Check sheet for the drawn part. Datum: minimum x, y, z corner. Units: mm. Give positions to 0.01 mm unless a question says otherwise; leave off trailing zeros. Loops run counter-clockwise (first coordinate to the right, second up) from the corner with the lowest first, then second, coordinate; pieces in that order, holes last. Notation, with made-up numbers: (-16, 63) - (36, 63) arc R17 ccw to (36, 78) - close; hole circle Ø1 at (66.5, 33.5). An arc over 180 degrees is marked (long way). One line per item, written item: value. Start each with the question number.
1. Gauge pin test, flat end, axial feed: pin 1 (0.8 mm diameter, centred on y = 1, z = 100, fed in from -X). Record the tip position at first contact, or that the pin passes through.
2. Scan lines: L1, parallel to Z at x = 14.5, y = 0.5; L2, parallel to X at y = 1.05, z = 121; L3, parallel to Z at x = 51.5, y = 1.4. Record each from-to range of solid material in increasing order. Write a range as [from, to].
3. Sectioned sample at D-D (z = 83). Record the cut outline in (x, y), plus the area to 3 significant figures.
4. Sectioned sample at B-B (y = 0.6). Record the cut outline in (x, z).
5. Sectioned sample at A-A (x = 50.5). Record the cut outline in (y, z).
6. Sectioned sample at C-C (z = 121). Record the cut outline in (x, y), plus the area to 3 significant figures.
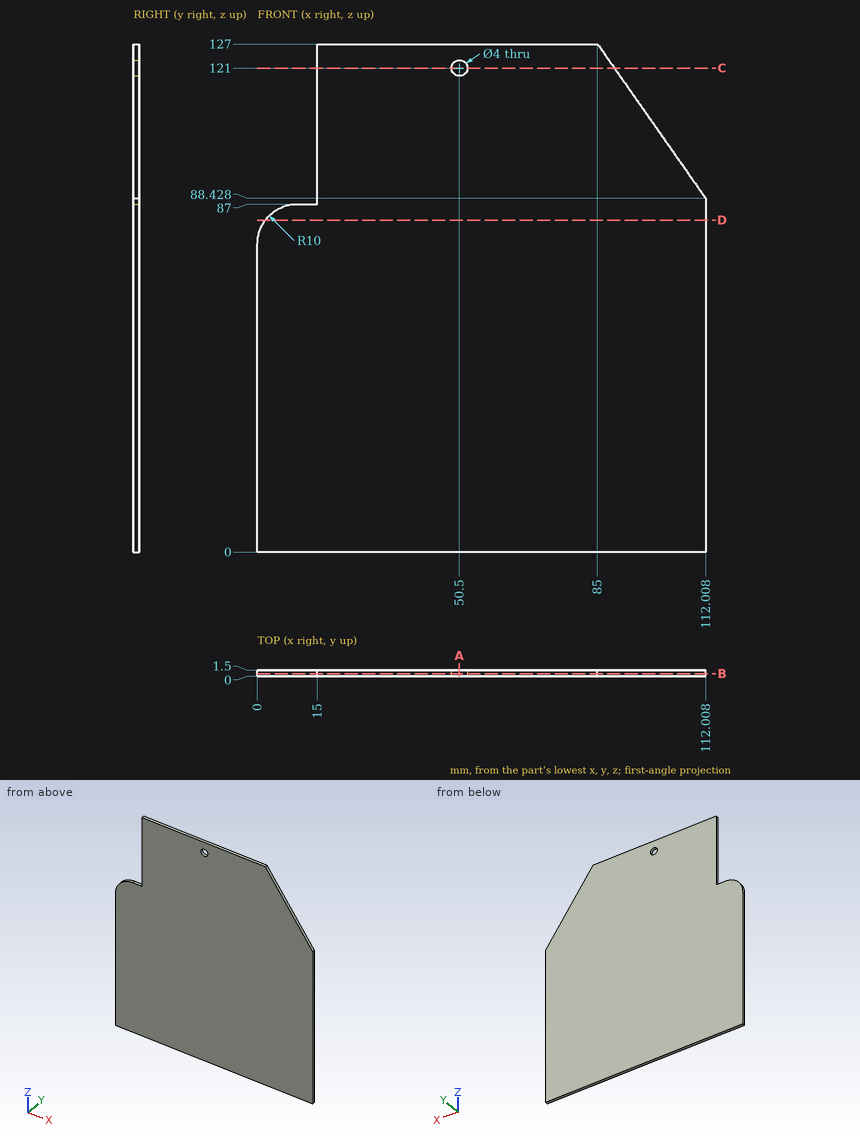
Results are:
1. pin 1: stops at x = 15
2. L1: z = [0, 87]
2. L2: x = [15, 48.5], [52.5, 89.2]
2. L3: z = [0, 119.27], [122.73, 127]
3. outline: (2, 0) - (112.01, 0) - (112.01, 1.5) - (2, 1.5) - close
3. area: 165 mm^2
4. outline: (0, 0) - (112.01, 0) - (112.01, 88.43) - (85, 127) - (15, 127) - (15, 87) - (10, 87) arc R10 ccw to (0, 77) - close; hole circle Ø4 at (50.5, 121)
5. outline: (0, 0) - (1.5, 0) - (1.5, 119) - (0, 119) - close; (0, 123) - (1.5, 123) - (1.5, 127) - (0, 127) - close
6. outline: (15, 0) - (48.5, 0) - (48.5, 1.5) - (15, 1.5) - close; (52.5, 0) - (89.2, 0) - (89.2, 1.5) - (52.5, 1.5) - close
6. area: 105 mm^2
